Geometry check sheet. Reference: the model listing, model coordinates, mm. Face numbers are marked on the shaded views. A direction names the side the tool comes from. Round coordinates to 2 decimals unless told otherwise and drop trailing zeros. Order: outer loops, then holes, each group sorted by start corner. A loop starts at its lowest first (then second) coordinate and runs counter-clockwise, first axis right, second up.
(1) Cross-section at A-A on x = 8.75. Enter the section's corners in (y, z).
(2) Draft check along Y on the marked faces 1, 2, 3 and 4. Enter one of: pulls with the +Y half, pulls with the -Y half, needs draft (parallel to the pull), parting line crosses it, or undercut.
(3) Cross-section at D-D on x = 6. Enter the section's corners in (y, z).
(4) Thickness scan on L1, parallel to Y at x = 4.25, z = 1.6; L2, parallel to X at y = 6, z = 1.1. Record the ranges inside material, lowest first.
(5) Set-up check for the marked faces 5 and 6: record each of +Z, -Z, +X, -X, +Y, -Y from which the full face is reachable in a straight line by a thin tool's end or side.
(6) Cross-section at B-B on z = 0.5. Enter the section's corners in (x, y), and give its area (3 significant figures).
(7) Gauge pin test, flat end, axial feed: P1, Ø0.5, axis at y = 11.5, z = 1.5, coming from the +X side. Record the tip position at first contact, or that the pin passes through.
(8) Cross-section at C-C on y = 8.75. Enter the section's corners in (x, z).
from build123d import *

# Parameters (mm, degrees)
F1_DEPTH   = 2
F2_SIZE2   = 1
F2_SIZE    = 0.2
F2_2_SIZE2 = 1
F2_2_SIZE  = 0.2
F2_3_SIZE2 = 1
F2_3_SIZE  = 0.2
F2_4_SIZE2 = 1
F2_4_SIZE  = 0.2
F3_SIZE2   = 0.2
F3_SIZE    = 1
F3_2_SIZE2 = 0.2
F3_2_SIZE  = 1
F3_3_SIZE2 = 0.2
F3_3_SIZE  = 1
F3_4_SIZE2 = 0.2
F3_4_SIZE  = 1


with BuildPart() as f1:
    # F0 (on Top) → F1 (new body)
    with BuildSketch(Plane.XY):
        Polygon((0, 13.7), (0, 0), (9, 0), (9, 1.5), (4, 1.5), (4, 3.2), (9, 3.2), (9, 4.7), (4, 4.7), (4, 9), (9, 9), (9, 10.5), (4, 10.5), (4, 12.2), (9, 12.2), (9, 13.7), (4, 13.7), align=None)
    extrude(amount=F1_DEPTH)

    # F2
    f2_edges = [f1.edges().sort_by_distance(p)[0] for p in [
        (9, 12.2, 1),
    ]]
    f2_side = f1.faces().sort_by_distance((9, 12.95, 1))[0]
    chamfer(f2_edges, length=F2_SIZE, length2=F2_SIZE2, reference=f2_side)

    # F2#2
    f2_2_edges = [f1.edges().sort_by_distance(p)[0] for p in [
        (9, 9, 1),
    ]]
    f2_2_side = f1.faces().sort_by_distance((9, 9.75, 1))[0]
    chamfer(f2_2_edges, length=F2_2_SIZE, length2=F2_2_SIZE2, reference=f2_2_side)

    # F2#3
    f2_3_edges = [f1.edges().sort_by_distance(p)[0] for p in [
        (9, 3.2, 1),
    ]]
    f2_3_side = f1.faces().sort_by_distance((9, 3.95, 1))[0]
    chamfer(f2_3_edges, length=F2_3_SIZE, length2=F2_3_SIZE2, reference=f2_3_side)

    # F2#4
    f2_4_edges = [f1.edges().sort_by_distance(p)[0] for p in [
        (9, 0, 1),
    ]]
    f2_4_side = f1.faces().sort_by_distance((9, 0.75, 1))[0]
    chamfer(f2_4_edges, length=F2_4_SIZE, length2=F2_4_SIZE2, reference=f2_4_side)

    # F3
    f3_edges = [f1.edges().sort_by_distance(p)[0] for p in [
        (9, 10.5, 1),
    ]]
    f3_side = f1.faces().sort_by_distance((6.5, 10.5, 1))[0]
    chamfer(f3_edges, length=F3_SIZE, length2=F3_SIZE2, reference=f3_side)

    # F3#2
    f3_2_edges = [f1.edges().sort_by_distance(p)[0] for p in [
        (9, 4.7, 1),
    ]]
    f3_2_side = f1.faces().sort_by_distance((6.5, 4.7, 1))[0]
    chamfer(f3_2_edges, length=F3_2_SIZE, length2=F3_2_SIZE2, reference=f3_2_side)

    # F3#3
    f3_3_edges = [f1.edges().sort_by_distance(p)[0] for p in [
        (9, 1.5, 1),
    ]]
    f3_3_side = f1.faces().sort_by_distance((6.5, 1.5, 1))[0]
    chamfer(f3_3_edges, length=F3_3_SIZE, length2=F3_3_SIZE2, reference=f3_3_side)

    # F3#4
    f3_4_edges = [f1.edges().sort_by_distance(p)[0] for p in [
        (9, 13.7, 1),
    ]]
    f3_4_side = f1.faces().sort_by_distance((4.5, 13.7, 1))[0]
    chamfer(f3_4_edges, length=F3_4_SIZE, length2=F3_4_SIZE2, reference=f3_4_side)


solid = f1.part
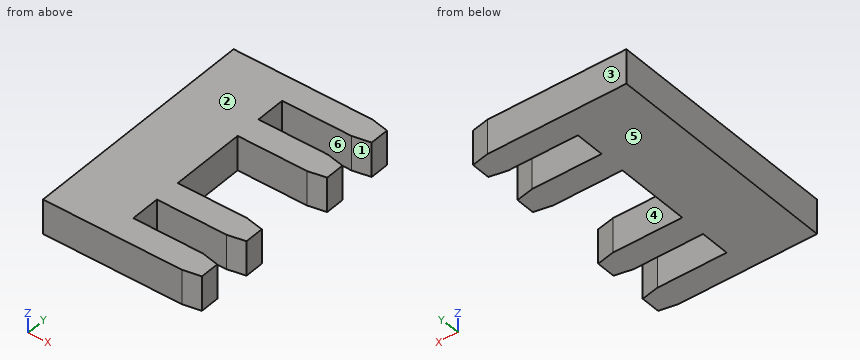
Found:
1. outline: (0.15, 0) - (1.35, 0) - (1.35, 2) - (0.15, 2) - close; (3.35, 0) - (4.55, 0) - (4.55, 2) - (3.35, 2) - close; (9.15, 0) - (10.35, 0) - (10.35, 2) - (9.15, 2) - close; (12.35, 0) - (13.55, 0) - (13.55, 2) - (12.35, 2) - close
2. face 1: undercut
2. face 2: needs draft
2. face 3: pulls with the +Y half
2. face 4: undercut
3. outline: (0, 0) - (1.5, 0) - (1.5, 2) - (0, 2) - close; (3.2, 0) - (4.7, 0) - (4.7, 2) - (3.2, 2) - close; (9, 0) - (10.5, 0) - (10.5, 2) - (9, 2) - close; (12.2, 0) - (13.7, 0) - (13.7, 2) - (12.2, 2) - close
4. L1: y = 0 to 1.5, 3.2 to 4.7, 9 to 10.5, 12.2 to 13.7
4. L2: x = 0 to 4
5. face 5: -Z, +X, -X, +Y, -Y
5. face 6: +Z, -Z, +X
6. outline: (0, 0) - (8, 0) - (9, 0.2) - (9, 1.3) - (8, 1.5) - (4, 1.5) - (4, 3.2) - (8, 3.2) - (9, 3.4) - (9, 4.5) - (8, 4.7) - (4, 4.7) - (4, 9) - (8, 9) - (9, 9.2) - (9, 10.3) - (8, 10.5) - (4, 10.5) - (4, 12.2) - (8, 12.2) - (9, 12.4) - (9, 13.5) - (8, 13.7) - (0, 13.7) - close
6. area: 84.0 mm2
7. P1: stops at x = 4
8. outline: (0, 0) - (4, 0) - (4, 2) - (0, 2) - close
